Could you check a few things on this drawing? It's one solid part, dimensions in mm from its lowest x, y, z. Give positions to 0.01 mm unless a question says otherwise; leave off trailing zeros. Write each loop counter-clockwise with the first axis right and the second up, starting at its lowest first coordinate (ties: lowest second). Pieces come first, ordered by that corner, then holes. Notation, with made-up numbers: M 18.5,-34 L 59.5,-34 A15 ccw 59.5,-18 Z; hole C 9.25,10.5 d8. An arc over 180 degrees is marked long. Write each question's results on one line, items separated by ' | '.
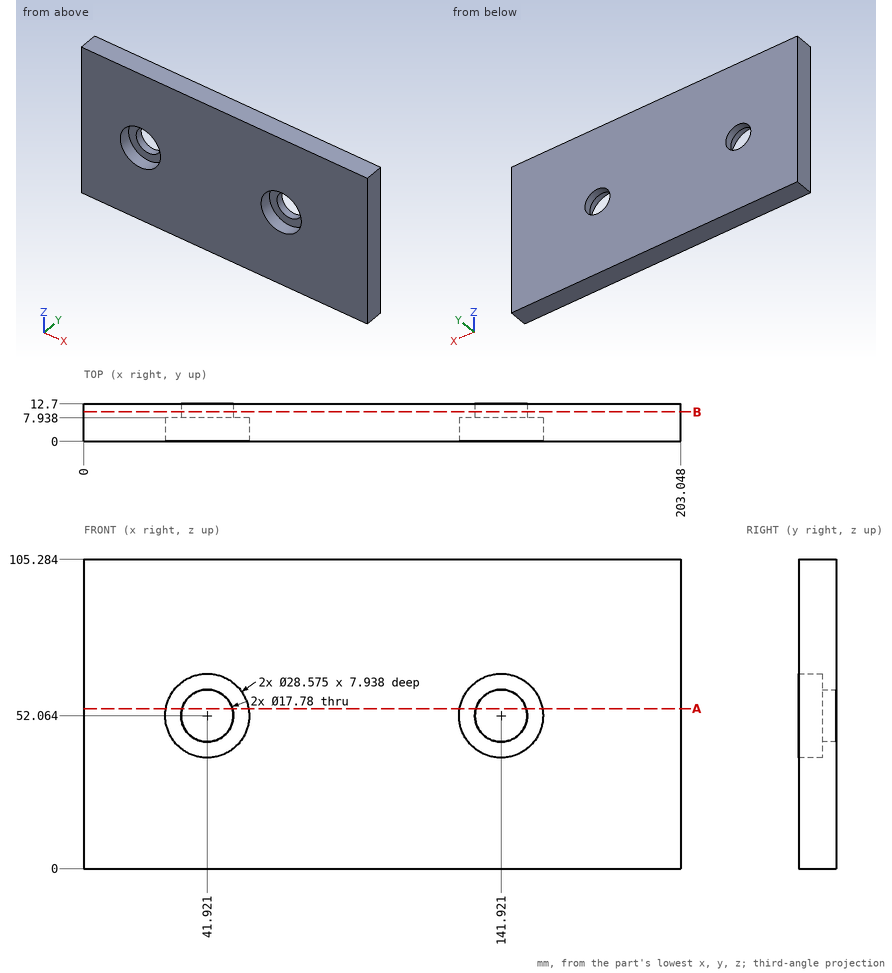
Item 1: I want a section at B-B, the plane y = 10. Please give me the cut outline in (x, z) (1 decimal).
Geometry says:
outline: M 0,0 L 203,0 L 203,105.3 L 0,105.3 Z; hole C 41.9,52.1 d17.8; hole C 141.9,52.1 d17.8
Item 2: If I drill on line 1 (X direction, y = 5, z = 57) (1 decimal); line 2 (Z direction, x = 142.5, y = 4.25) (1 decimal); line 3 (Z direction, x = 51, y = 5.25) (1 decimal), over which ranges is the centre line in solid material (lowest first)? Write a range as from..to.
Geometry says:
line 1: x = 0..28.5, 55.3..128.5, 155.3..203 | line 2: z = 0..37.8, 66.3..105.3 | line 3: z = 0..41, 63.1..105.3
Item 3: I'm going to push flat-ended pins straight in: pin 1 (10 mm diameter, centred on x = 83.5, z = 31, fed in from -Y); pin 2 (23 mm diameter, centred on x = 41.92, z = 52.06, fed in from -Y); pin 3 (14 mm diameter, centred on x = 141.92, z = 52.06, fed in from -Y). Where does each tip first touch, or does it pass through?
Geometry says:
pin 1: stops at y = 0 | pin 2: stops at y = 7.94 | pin 3: passes through
Item 4: I want a section at A-A, the plane z = 54.5. Please give me the cut outline in (x, y), and give its area (3 significant figures).
Geometry says:
outline: M 0,0 L 27.84,0 L 27.84,7.94 L 33.37,7.94 L 33.37,12.7 L 0,12.7 Z; M 50.47,7.94 L 56,7.94 L 56,0 L 127.84,0 L 127.84,7.94 L 133.37,7.94 L 133.37,12.7 L 50.47,12.7 Z; M 150.47,7.94 L 156,7.94 L 156,0 L 203.05,0 L 203.05,12.7 L 150.47,12.7 Z | area: 1,970 mm2
